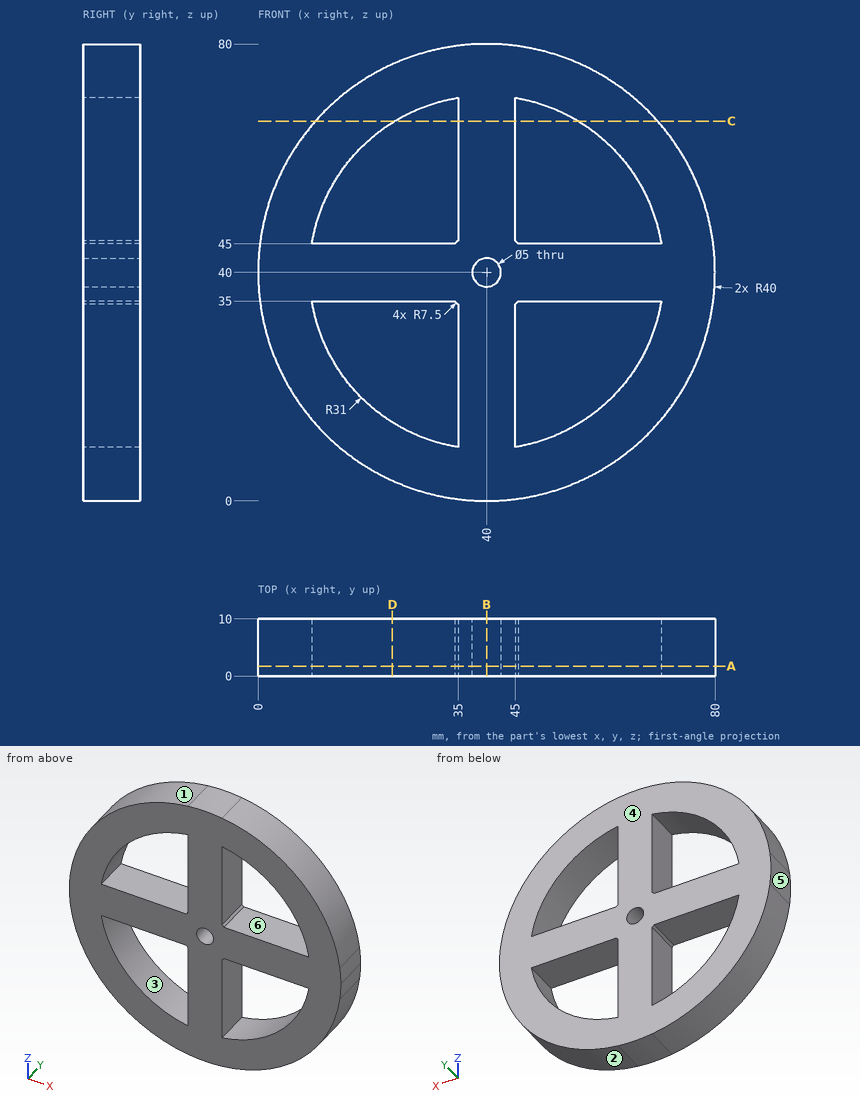
Could you check a few things on this drawing? It's one solid part, dimensions in mm from its lowest x, y, z. A direction names the side the tool comes from. Give positions to 0.01 mm unless a question says otherwise; leave off trailing zeros. Loops run counter-clockwise (first coordinate to the right, second up) from the corner with the lowest first, then second, coordinate; pieces in that order, holes last. Notation, with made-up numbers: M -13,-14.5 L 4,-14.5 A19 cw 4,19.5 Z; hole C 54,-15.5 d1. An arc over 180 degrees is marked long. One line per question, with ' | ' between items. Start each with the question number.
Q1. If we section it at C-C (z = 66.5): Please give me the cut outline in (x, y).
Q2. If we mould it in two halves opening along X, with no side actions, what happens to the marked faces 1, 2, 3 and 4? For each: +X half, -X half, draft (parallel to the pull), parting line (faces both ways), or undercut.
Q3. If we section it at D-D (x = 23.5): Please give me the cut outline in (y, z), plus the area to 3 significant figures.
Q4. If we section it at B-B (x = 40): Please give me the cut outline in (y, z), plus the area to 3 significant figures.
Q5. If we section it at A-A (y = 1.75): Please give me the cut outline in (x, z), plus the area to 3 significant figures.
Q6. If I drill on line 1 (Z direction, x = 40, y = 5.5); line 2 (Z direction, x = 53.5, y = 7.25); line 3 (Z direction, x = 63.5, y = 2.5), over which ranges is the centre line in solid material (lowest first)? Write a range as from..to.
Q7. For the marked faces 5 and 6, which set-ups out of +Z, -Z, +X, -X, +Y, -Y let a thin tool reach every point of the face, with its end or its side?
Q8. For pin 1 Ø5 at (x, y) = (16.5, 5) entering from +Z; pin 2 Ø1.5 at (y, z) = (8.5, 31.5) entering from -X; pin 3 Ø1.5 at (y, z) = (5.5, 25.5) entering from -X, each with a flat end and sliding along its axis, tell me the tip position at first contact or that it passes through.
Computed:
1) outline: M 10.04,0 L 23.91,0 L 23.91,10 L 10.04,10 Z; M 35,0 L 45,0 L 45,10 L 35,10 Z; M 56.09,0 L 69.96,0 L 69.96,10 L 56.09,10 Z
2) face 1: -X half | face 2: +X half | face 3: undercut | face 4: draft
3) outline: M 0,3.56 L 10,3.56 L 10,13.76 L 0,13.76 Z; M 0,35 L 10,35 L 10,45 L 0,45 Z; M 0,66.24 L 10,66.24 L 10,76.44 L 0,76.44 Z | area: 304 mm²
4) outline: M 0,0 L 10,0 L 10,37.5 L 0,37.5 Z; M 0,42.5 L 10,42.5 L 10,80 L 0,80 Z | area: 750 mm²
5) outline: M 0.31,35 A40 ccw 35,0.31 A40 ccw 45,0.31 A40 ccw 79.69,35 A40 ccw 80,40 A40 ccw 79.69,45 A40 ccw 45,79.69 A40 ccw 35,79.69 A40 ccw 0.31,45 A40 ccw Z; hole M 9.41,35 A31 ccw 35,9.41 L 35,34.41 A7.5 cw 34.41,35 Z; hole M 9.41,45 L 34.41,45 A7.5 cw 35,45.59 L 35,70.59 A31 ccw Z; hole C 40,40 d5; hole M 45,9.41 A31 ccw 70.59,35 L 45.59,35 A7.5 cw 45,34.41 Z; hole M 45,45.59 A7.5 cw 45.59,45 L 70.59,45 A31 ccw 45,70.59 Z | area: 3,120 mm²
6) line 1: z = 0..37.5, 42.5..80 | line 2: z = 2.35..12.09, 35..45, 67.91..77.65 | line 3: z = 7.63..19.78, 35..45, 60.22..72.37
7) face 5: -X, +Y, -Y | face 6: +Y, -Y
8) pin 1: stops at z = 74.04 | pin 2: stops at x = 0.76 | pin 3: stops at x = 2.44
